Check sheet for the modelled part. Datum: model origin and axes. Units: mm. A direction names the side the tool comes from. Round coordinates to 2 decimals unless told otherwise and drop trailing zeros. Loops run counter-clockwise (first coordinate to the right, second up) from the corner with the lowest first, then second, coordinate; pieces in that order, holes last. Notation, with made-up numbers: M 9.25,58 L 44.25,58 A6 cw 44.25,69 Z; hole C -31,-15 d6. An arc over 180 degrees is marked long. Write item = value, one per line. Start each with the question number.
(1) Scan lines: L1, parallel to X at y = 5.75, z = 30; L2, parallel to X at y = 4, z = -43.5; L3, parallel to Y at x = -32.5, z = -5.5. Record each from-to range of solid material in increasing order. Write a range as from..to.
(2) Mould release check, pull along Y, two halves, no side actions. Record for faces 1 (the face through (1, 6, -32)), 2 (the face through (-63.2, 2.6, -59.033)), 3 (the face through (27.56, 14.31, -49.03)): pulls with the +Y half, pulls with the -Y half, needs draft (parallel to the pull), parting line crosses it, or undercut.
(3) Set-up check for faces 4 (the face through (-96, 1, -5.033)), 5 (the face through (27.561, 9.811, -55.275)), 6 (the face through (24.519, 9, -47)): record each of +Z, -Z, +X, -X, +Y, -Y from which the full face is reachable in a straight line by a thin tool's end or side.
(4) Go/stop test with flat-tipped pins: P1, Ø2.5, axis at y = 1.5, z = 23.5, coming from the -X side; P2, Ø3.5, axis at x = 3.52, z = -32.03, coming from the +Y side; P3, Ø0.9, axis at x = -97.5, y = 2, coming from the +Z side; P4, Ø10, axis at x = -14.5, z = 26.5, coming from the +Y side. Record where each tip stops, or that it passes through.
(5) Cross-section at A-A on z = -40. Record the boundary of the cut face in (x, y).
(6) Cross-section at C-C on z = 15. Record the boundary of the cut face in (x, y), plus the area to 3 significant figures.
(7) Cross-section at B-B on x = -37. Record the boundary of the cut face in (y, z).
from build123d import *

# Parameters (mm, degrees)
SKETCH1_R                       = 2
BOSS_EXTRUDE1_DEPTH             = 3
SKETCH4_R                       = 3
SKETCH4_R_2                     = 2
BOSS_EXTRUDE2_DEPTH             = 3
CHAMFER1_SIZE                   = 3
BOSS_EXTRUDE3_DEPTH             = 4
BOSS_EXTRUDE4_DEPTH             = 20
CUT_EXTRUDE1_REACH              = 168.064
F_4_0MM_DOWEL_HOLE1_D           = 4
F_4_0MM_DOWEL_HOLE1_CSINK_D     = 4.05
F_4_0MM_DOWEL_HOLE1_CSINK_ANGLE = 90
SKETCH13_R                      = 2
BOSS_EXTRUDE5_DEPTH             = 6


with BuildPart() as part:
    # Sketch1 → Boss-Extrude1 (new body)
    with BuildSketch(Plane(origin=(0, 0, 0), x_dir=(1, 0, 0), z_dir=(0, 1, 0))):
        with BuildLine():
            ThreePointArc((-123.480593783, 26.275205138), (-122.719389108, 22.448370814), (-120.551661595, 19.204137326))
            Line((-120.551661595, 19.204137326), (-109.309020908, 7.961496639))
            ThreePointArc((-109.309020908, 7.961496639), (-106.064787419, 5.793769125), (-102.237953096, 5.032564451))
            Line((-102.237953096, 5.032564451), (-90.522224343, 5.032564451))
            ThreePointArc((-90.522224343, 5.032564451), (-86.69539002, 4.271359776), (-83.451156531, 2.103632262))
            Line((-83.451156531, 2.103632262), (-82.409525971, 1.062001702))
            ThreePointArc((-82.409525971, 1.062001702), (-80.241798458, -2.182231786), (-79.480593783, -6.00906611))
            Line((-79.480593783, -6.00906611), (-79.480593783, -32.967435549))
            ThreePointArc((-79.480593783, -32.967435549), (-76.551661595, -40.038503361), (-69.480593783, -42.967435549))
            Line((-69.480593783, -42.967435549), (30.519406217, -42.967435549))
            Line((30.519406217, -42.967435549), (30.519406217, 59.032564451))
            Line((30.519406217, 59.032564451), (-123.480593783, 59.032564451))
            Line((-123.480593783, 59.032564451), (-123.480593783, 26.275205138))
        make_face()
        with Locations((-105.480593783, 32.032564451)):
            Circle(SKETCH1_R, mode=Mode.SUBTRACT)
        with Locations((3.519406217, 32.032564451)):
            Circle(SKETCH1_R, mode=Mode.SUBTRACT)
        with Locations((15.519406217, -30.967435549)):
            Circle(SKETCH1_R, mode=Mode.SUBTRACT)
    extrude(amount=BOSS_EXTRUDE1_DEPTH)

    # Sketch4 → Boss-Extrude2 (add)
    # profile 1 of 3: a face of its own
    with BuildSketch(Plane(origin=(0, 3, 0), x_dir=(1, 0, 0), z_dir=(0, 1, 0))):
        with Locations(Location((-105.480593783, 32.032564451, 0), (0, 0, 90))):
            Circle(SKETCH4_R)
        with Locations(Location((-105.480593783, 32.032564451, 0), (0, 0, 270))):
            Circle(SKETCH4_R_2, mode=Mode.SUBTRACT)
    # profile 2 of 3: a face of its own
    with BuildSketch(Plane(origin=(0, 3, 0), x_dir=(1, 0, 0), z_dir=(0, 1, 0))):
        with Locations(Location((15.519406217, -30.967435549, 0), (0, 0, 90))):
            Circle(SKETCH4_R)
        with Locations(Location((15.519406217, -30.967435549, 0), (0, 0, 270))):
            Circle(SKETCH4_R_2, mode=Mode.SUBTRACT)
    # profile 3 of 3: a face of its own
    with BuildSketch(Plane(origin=(0, 3, 0), x_dir=(1, 0, 0), z_dir=(0, 1, 0))):
        with Locations(Location((3.519406217, 32.032564451, 0), (0, 0, 90))):
            Circle(SKETCH4_R)
        with Locations(Location((3.519406217, 32.032564451, 0), (0, 0, 270))):
            Circle(SKETCH4_R_2, mode=Mode.SUBTRACT)
    extrude(amount=BOSS_EXTRUDE2_DEPTH)

    # Chamfer1
    chamfer1_edges = [part.edges().sort_by_distance(p)[0] for p in [
        (-105.480593783, 3, -29.032564451),
        (15.519406217, 3, 33.967435549),
        (3.519406217, 3, -29.032564451),
    ]]
    chamfer(chamfer1_edges, length=CHAMFER1_SIZE - 0.0001)  # a hair under: the kernel refuses the full size

    # Sketch7 → Boss-Extrude3 (add)
    with BuildSketch(Plane(origin=(0, 0, -59.032564451), x_dir=(-1, 0, 0), z_dir=(0, 0, -1))):
        with BuildLine():
            Line((113.480593783, 14.4), (113.480593783, 3))
            Line((113.480593783, 3), (123.480593783, 3))
            Line((123.480593783, 3), (123.480593783, 14.4))
            ThreePointArc((123.480593783, 14.4), (118.480593783, 19.4), (113.480593783, 14.4))
        make_face()
    extrude(amount=-BOSS_EXTRUDE3_DEPTH)

    # Sketch9 → Boss-Extrude4 (add)
    with BuildSketch(Plane.XY.offset(-55.032564451)):
        with BuildLine():
            Line((-123.480593783, 3), (-113.480593783, 3))
            Line((-113.480593783, 3), (-113.480593783, 14.4))
            ThreePointArc((-113.480593783, 14.4), (-118.480593783, 19.4), (-123.480593783, 14.4))
            Line((-123.480593783, 14.4), (-123.480593783, 3))
        make_face()
    extrude(amount=BOSS_EXTRUDE4_DEPTH)

    # Sketch10 → Cut-Extrude1 (cut, up to next)
    with BuildSketch(Plane.ZY.offset(123.480593783), mode=Mode.PRIVATE) as cut_extrude1_sk1:
        Polygon((-53.032564451, 19.4), (-36.632564451, 3), (-35.032564451, 3), (-35.032564451, 19.4), align=None)
    cut_extrude1_tool1 = extrude(cut_extrude1_sk1.sketch, amount=-CUT_EXTRUDE1_REACH, mode=Mode.PRIVATE) & part.part
    add(cut_extrude1_tool1.solids().sort_by_distance((-123.480594, 13.487075, -41.076102))[0], mode=Mode.SUBTRACT)

    # Ø4.0mm Dowel Hole1 (through all)
    with Locations(Plane(origin=(0, 0, -59.032564451), x_dir=(-1, 0, 0), z_dir=(0, 0, -1))):
        with Locations((118.480593783, 14.4)):
            CounterSinkHole(F_4_0MM_DOWEL_HOLE1_D / 2, F_4_0MM_DOWEL_HOLE1_CSINK_D / 2, counter_sink_angle=F_4_0MM_DOWEL_HOLE1_CSINK_ANGLE)

    # Sketch13 → Boss-Extrude5 (add)
    # profile 1 of 2: a face of its own
    with BuildSketch(Plane(origin=(30.519406217, 0, 0), x_dir=(0, 0, -1), z_dir=(1, 0, 0))):
        with BuildLine():
            Line((-26.589524244, 16.815345234), (-18.967435549, 3))
            Line((-18.967435549, 3), (-42.967435549, 3))
            Line((-42.967435549, 3), (-35.345346855, 16.815345234))
            ThreePointArc((-35.345346855, 16.815345234), (-30.967435549, 19.4), (-26.589524244, 16.815345234))
        make_face()
        with Locations((-30.967435549, 14.4)):
            Circle(SKETCH13_R, mode=Mode.SUBTRACT)
    # profile 2 of 2: a face of its own
    with BuildSketch(Plane(origin=(30.519406217, 0, 0), x_dir=(0, 0, -1), z_dir=(1, 0, 0))):
        with BuildLine():
            Line((59.032564451, 3), (51.410475756, 16.815345234))
            ThreePointArc((51.410475756, 16.815345234), (47.032564451, 19.4), (42.654653145, 16.815345234))
            Line((42.654653145, 16.815345234), (35.032564451, 3))
            Line((35.032564451, 3), (59.032564451, 3))
        make_face()
        with Locations(Location((47.032564451, 14.4, 0), (0, 0, 180))):
            Circle(SKETCH13_R, mode=Mode.SUBTRACT)
    extrude(amount=-BOSS_EXTRUDE5_DEPTH)


solid = part.part
Result:
q1.L1 = 12.42..13.77, 17.27..18.62, 24.52..30.52
q1.L2 = -123.48..-113.48, 24.52..30.52
q1.L3 = 0..3
q2.face_1 = pulls with the +Y half
q2.face_2 = needs draft
q2.face_3 = undercut
q3.face_4 = +Z, -X, +Y, -Y
q3.face_5 = -Z, +X, +Y
q3.face_6 = +Z, -Z, +Y
q4.P1 = -79.48
q4.P2 = through
q4.P3 = -5.03
q4.P4 = 3
q5.outline = M -123.48,0 L 30.52,0 L 30.52,12 L 24.52,12 L 24.52,3 L -113.48,3 L -113.48,6.37 L -123.48,6.37 Z
q6.outline = M -79.48,0 L 30.52,0 L 30.52,3 L -79.48,3 Z
q6.area = 330 mm^2
q7.outline = M 0,-59.03 L 3,-59.03 L 3,42.97 L 0,42.97 Z
